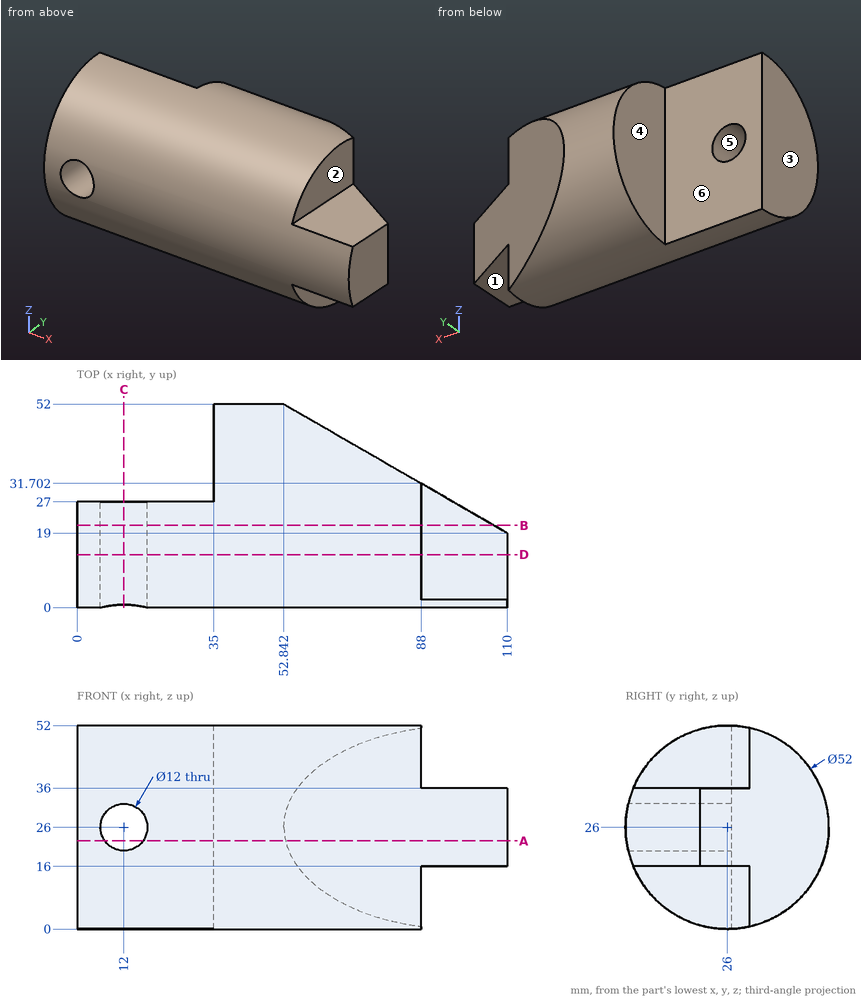
Check sheet for the drawn part. Datum: minimum x, y, z corner. Units: mm. A direction names the side the tool comes from. Round coordinates to 2 decimals unless told otherwise and drop trailing zeros. Write each loop counter-clockwise with the first axis right and the second up, starting at its lowest first coordinate (ties: lowest second). Pieces come first, ordered by that corner, then holes. Notation, with made-up numbers: (-27.5, 25.5) -> (6.5, 25.5) arc R28 ccw to (6.5, 58.5) -> close; hole circle Ø9 at (60.5, 83.5). An arc over 180 degrees is marked (long way). Write each question's results on one line, items separated by ' | '. Start each with the question number.
1. Cross-section at C-C (x = 12). Enter the section's corners in (y, z).
2. Draft check along X on the marked faces 4, 5 and 6. Enter one of: +X half, -X half, draft (parallel to the pull), parting line (faces both ways), or undercut.
3. Depth check by flat-ended pin: P1, Ø7.5, axis at y = 37.5, z = 33.5, coming from the -X side; P2, Ø3, axis at x = 87, y = 13.5, coming from the -Z side; P3, Ø11, axis at x = 98.5, y = 16.5, coming from the +Z side. Enter the tip coordinate at first touch or a pass-through.
4. Material ranges on probe 1 along Z at (x, y) = (94.5, 14.5); probe 2 along X at (y, z) = (23, 22.5) (1 decimal); probe 3 along X at (y, z) = (29, 38), recorded low to high. Write a range as from..to.
5. Cross-section at A-A (z = 22.5). Enter the section's corners in (x, y).
6. Set-up check for the marked faces 1, 2 and 3: record each of +Z, -Z, +X, -X, +Y, -Y from which the full face is reachable in a straight line by a thin tool's end or side.
7. Cross-section at B-B (y = 21). Enter the section's corners in (x, z) (1 decimal).
8. Cross-section at D-D (y = 13.5). Enter the section's corners in (x, z), then the cut area to 3 significant figures.
Solutions:
1) outline: (0.7, 20) arc R26 ccw to (27, 0.02) -> (27, 20) -> close; (0.7, 32) -> (27, 32) -> (27, 51.98) arc R26 ccw to start
2) face 4: -X half | face 5: undercut | face 6: draft
3) P1: stops at x = 35 | P2: stops at z = 2.44 | P3: stops at z = 36
4) probe 1: z = 16..36 | probe 2: x = 0..7.1, 16.9..103.1 | probe 3: x = 35..88
5) outline: (0, 0.24) -> (7.13, 0.24) -> (7.13, 27) -> (0, 27) -> close; (16.87, 0.24) -> (110, 0.24) -> (110, 19) -> (53.25, 51.76) -> (35, 51.76) -> (35, 27) -> (16.87, 27) -> close
6) face 1: -Z, +X, +Y, -Y | face 2: +Z, +X, +Y, -Y | face 3: +Z, -Z, -X, +Y, -Y
7) outline: (0, 0.5) -> (88, 0.5) -> (88, 16) -> (106.5, 16) -> (106.5, 36) -> (88, 36) -> (88, 51.5) -> (0, 51.5) -> close; hole circle Ø12 at (12, 26)
8) outline: (0, 3.2) -> (88, 3.2) -> (88, 16) -> (110, 16) -> (110, 36) -> (88, 36) -> (88, 48.8) -> (0, 48.8) -> close; hole circle Ø12 at (12, 26) | area: 4,340 mm2
